Geometry check sheet. Reference: the model listing, model coordinates, mm. A direction names the side the tool comes from. Round coordinates to 2 decimals unless told otherwise and drop trailing zeros. Answer as CSV lines item,"result". Start each with the question number.
1) Access from +Z, -Z, +X, -X, +Y, -Y to the whole of each face (thin tool, end or side, straight path). Record for faces 1 (the flat face through (2, -4, -130)), 2 (the flat face through (70, -4, 0)).
2) Thickness scan on line 1 along Z through (x, y) = (139.5, -6); line 2 along X through (y, z) = (-7, 15); line 3 along X through (y, z) = (-6.25, -100). Record the ranges inside material, lowest first.
3) Cross-section at A-A on y = -3.25. State how many separate pieces and enclosed holes the cut face has, and give its area (3 significant figures).
4) Depth check by flat-ended pin: P1, Ø3, axis at x = -140, z = 34.5, coming from the +Y side. Enter the tip coordinate at first touch or a pass-through.
5) Draft check along Z on faces 3 (the flat face through (-2, -9, -2)), 4 (the flat face through (-2, -4, 130)), 5 (the flat face through (160, -4, 1)). Enter one of: released by +Z, released by -Z, zero draft, split by the parting line, or undercut.
from build123d import *

# Parameters (mm, degrees)
ESQUISSE3_R                  = 2.1
BOSS_EXTRU_2_DEPTH           = 9
ESQUISSE4_R                  = 3.05
ENL_V_MAT_EXTRU_3_DEPTH      = 5
ESQUISSE5_R                  = 2.05
ENL_V_MAT_EXTRU_4_DEPTH      = 215.198506064
ENL_V_MAT_EXTRU_5_DEPTH      = 215.198506064
ENL_V_MAT_EXTRU_5_DEPTH_BACK = 215.198506064
ESQUISSE6_R                  = 2.05
ESQUISSE7_R                  = 2.05
ENL_V_MAT_EXTRU_6_DEPTH      = 215.198506064


with BuildPart() as part:
    # Esquisse3 → Boss.-Extru.2 (new body)
    with BuildSketch(Plane(origin=(0, 0, 0), x_dir=(1, 0, 0), z_dir=(0, 1, 0))):
        Polygon((155, 130), (-155, 130), (-170, 115), (-170, -115), (-155, -130), (155, -130), (170, -115), (170, 115), align=None)
        with Locations(Location((-140, 100, 0), (0, 0, 270))):
            Circle(ESQUISSE3_R, mode=Mode.SUBTRACT)
        with Locations(Location((-140, -100, 0), (0, 0, 90))):
            Circle(ESQUISSE3_R, mode=Mode.SUBTRACT)
        with Locations(Location((140, -100, 0), (0, 0, 270))):
            Circle(ESQUISSE3_R, mode=Mode.SUBTRACT)
        with Locations(Location((140, 100, 0), (0, 0, 90))):
            Circle(ESQUISSE3_R, mode=Mode.SUBTRACT)
        with BuildLine():
            Line((-160, -46), (-160, 46))
            ThreePointArc((-160, 46), (-158.828427125, 48.828427125), (-156, 50))
            Line((-156, 50), (-149, 50))
            ThreePointArc((-149, 50), (-146.171572875, 48.828427125), (-145, 46))
            Line((-145, 46), (-145, -46))
            ThreePointArc((-145, -46), (-146.171572875, -48.828427125), (-149, -50))
            Line((-149, -50), (-156, -50))
            ThreePointArc((-156, -50), (-158.828427125, -48.828427125), (-160, -46))
        make_face(mode=Mode.SUBTRACT)
        with BuildLine():
            Line((-105, 0), (-105, 31))
            ThreePointArc((-105, 31), (-103.828427125, 33.828427125), (-101, 35))
            Line((-101, 35), (-74, 35))
            ThreePointArc((-74, 35), (-71.171572875, 33.828427125), (-70, 31))
            Line((-70, 31), (-70, -31))
            ThreePointArc((-70, -31), (-71.171572875, -33.828427125), (-74, -35))
            Line((-74, -35), (-101, -35))
            ThreePointArc((-101, -35), (-103.828427125, -33.828427125), (-105, -31))
            Line((-105, -31), (-105, 0))
        make_face(mode=Mode.SUBTRACT)
        with BuildLine():
            Line((156, 50), (149, 50))
            ThreePointArc((149, 50), (146.171572875, 48.828427125), (145, 46))
            Line((145, 46), (145, -46))
            ThreePointArc((145, -46), (146.171572875, -48.828427125), (149, -50))
            Line((149, -50), (156, -50))
            ThreePointArc((156, -50), (158.828427125, -48.828427125), (160, -46))
            Line((160, -46), (160, 46))
            ThreePointArc((160, 46), (158.828427125, 48.828427125), (156, 50))
        make_face(mode=Mode.SUBTRACT)
        with BuildLine():
            Line((105, 0), (105, 31))
            ThreePointArc((105, 31), (103.828427125, 33.828427125), (101, 35))
            Line((101, 35), (74, 35))
            ThreePointArc((74, 35), (71.171572875, 33.828427125), (70, 31))
            Line((70, 31), (70, -31))
            ThreePointArc((70, -31), (71.171572875, -33.828427125), (74, -35))
            Line((74, -35), (101, -35))
            ThreePointArc((101, -35), (103.828427125, -33.828427125), (105, -31))
            Line((105, -31), (105, 0))
        make_face(mode=Mode.SUBTRACT)
    extrude(amount=-BOSS_EXTRU_2_DEPTH)

    # Esquisse4 → Enlèv. mat.-Extru.3 (cut)
    with BuildSketch(Plane(origin=(0, 0, 0), x_dir=(1, 0, 0), z_dir=(0, 1, 0))):
        with Locations(Location((-139.5, 33.5, 0), (0, 0, 270))):
            Circle(ESQUISSE4_R)
        with Locations(Location((-139.5, -33.5, 0), (0, 0, 90))):
            Circle(ESQUISSE4_R)
        with Locations(Location((139.5, -33.5, 0), (0, 0, 270))):
            Circle(ESQUISSE4_R)
        with Locations(Location((139.5, 33.5, 0), (0, 0, 90))):
            Circle(ESQUISSE4_R)
    extrude(amount=-ENL_V_MAT_EXTRU_3_DEPTH, mode=Mode.SUBTRACT)

    # Esquisse5 → Enlèv. mat.-Extru.4 (cut, through all)
    with BuildSketch(Plane(origin=(0, 0, 0), x_dir=(1, 0, 0), z_dir=(0, 1, 0))):
        with Locations(Location((-139.5, 60, 0), (0, 0, 270))):
            Circle(ESQUISSE5_R)
        with Locations(Location((-139.5, -60, 0), (0, 0, 90))):
            Circle(ESQUISSE5_R)
        with Locations(Location((139.5, -60, 0), (0, 0, 270))):
            Circle(ESQUISSE5_R)
        with Locations(Location((139.5, 60, 0), (0, 0, 90))):
            Circle(ESQUISSE5_R)
    extrude(amount=-ENL_V_MAT_EXTRU_4_DEPTH, mode=Mode.SUBTRACT)

    # Esquisse6 → Enlèv. mat.-Extru.5 (cut, two sides: drawn at the far end of the back side and taken through both)
    with BuildSketch(Plane(origin=(0, 0, 0), x_dir=(1, 0, 0), z_dir=(0, 1, 0)).offset(-ENL_V_MAT_EXTRU_5_DEPTH_BACK)):
        with Locations(Location((-65, 25.5, 0), (0, 0, 270))):
            Circle(ESQUISSE6_R)
        with Locations(Location((-48.3, 25.5, 0), (0, 0, 270))):
            Circle(ESQUISSE6_R)
        with Locations(Location((-48.3, -25.5, 0), (0, 0, 270))):
            Circle(ESQUISSE6_R)
        with Locations(Location((-65, -25.5, 0), (0, 0, 270))):
            Circle(ESQUISSE6_R)
        with Locations(Location((65, -25.5, 0), (0, 0, 270))):
            Circle(ESQUISSE6_R)
        with Locations(Location((48.3, -25.5, 0), (0, 0, 270))):
            Circle(ESQUISSE6_R)
        with Locations(Location((48.3, 25.5, 0), (0, 0, 270))):
            Circle(ESQUISSE6_R)
        with Locations(Location((65, 25.5, 0), (0, 0, 270))):
            Circle(ESQUISSE6_R)
    extrude(amount=ENL_V_MAT_EXTRU_5_DEPTH + ENL_V_MAT_EXTRU_5_DEPTH_BACK, mode=Mode.SUBTRACT)

    # Esquisse7 → Enlèv. mat.-Extru.6 (cut, through all)
    with BuildSketch(Plane(origin=(0, 0, 0), x_dir=(1, 0, 0), z_dir=(0, 1, 0))):
        with Locations(Location((0, 100, 0), (0, 0, 270))):
            Circle(ESQUISSE7_R)
        with Locations(Location((0, -100, 0), (0, 0, 90))):
            Circle(ESQUISSE7_R)
    extrude(amount=-ENL_V_MAT_EXTRU_6_DEPTH, mode=Mode.SUBTRACT)


solid = part.part
Answer block:
1,face 1,"-Z, +X, -X, +Y, -Y"
1,face 2,"+Y, -Y"
2,line 1,"z = -130 to -102.04, -97.96 to -62.05, -57.95 to 57.95, 62.05 to 97.96, 102.04 to 130"
2,line 2,"x = -170 to -160, -145 to -105, -70 to 70, 105 to 145, 160 to 170"
2,line 3,"x = -170 to -142.1, -137.9 to -2.05, 2.05 to 137.9, 142.1 to 170"
3,separate pieces,"1"
3,enclosed holes,"26"
3,area,"79,700 mm^2"
4,P1,"stops at y = -5"
5,face 3,"zero draft"
5,face 4,"released by +Z"
5,face 5,"undercut"
